```python
from build123d import *


with BuildPart() as part:
    # Sketch1 → Revolve1 (revolve)
    with BuildSketch(Plane.XY, mode=Mode.PRIVATE) as revolve1_sk:
        Polygon((-52, 0), (-52, 2), (-42, 2), (-42, 3), (42, 3), (42, 2), (52, 2), (52, 0), align=None)
    revolve(revolve1_sk.sketch.rotate(Axis((-52, 0, 0), (1, 0, 0)), 180), axis=Axis((-52, 0, 0), (1, 0, 0)))  # turned: the seam where the file's is


solid = part.part
```
Work out the finished part from the listing and answer in its coordinate system (mm). A direction names the side the tool comes from. Round coordinates to 2 decimals unless told otherwise and drop trailing zeros. Loops run counter-clockwise (first coordinate to the right, second up) from the corner with the lowest first, then second, coordinate; pieces in that order, holes last. Notation, with made-up numbers: (10, 8.25) -> (55, 8.25) arc R14 ccw to (55, 14.25) -> close; hole circle Ø8 at (-12.75, 32.5). An arc over 180 degrees is marked (long way). Write each question's results on one line, items separated by ' | '. Start each with the question number.
1. Section C-C (x = 7.5) is taken. Determine the outline of the cut face in (y, z), plus the area to 3 significant figures.
2. Find the intervals of material crossed by probe 1 along Y at (x, z) = (32.5, 0.1); probe 2 along X at (y, z) = (-2.25, 0.95); probe 3 along Y at (x, z) = (35.5, -2.4), in increasing order. Write a range as from..to.
3. Section A-A (y = 0) is taken. Determine the outline of the cut face in (x, z).
4. A tool of negligible diameter and unlimited length cuts with its end or side. For faces 1 (the face through (-47, 0, 2)), 2 (the face through (42, -1, 2)), 3 (the face through (-52, 0, 0)), from which of +Z, -Z, +X, -X, +Y, -Y can it reach the whole face along a straight path? Write none if from no direction.
5. Given pin 1 Ø2 at (x, y) = (31, 1.5) entering from -Z; pin 2 Ø1.5 at (x, z) = (-34, 2) entering from -Y; pin 3 Ø1 at (y, z) = (-0.5, -2.5) entering from -X; pin 4 Ø1.5 at (x, z) = (29, -0.5) entering from -Y, each flat-ended and moving along its own axis, determine where each tip first touches the part or whether it passes through.
6. Section D-D (x = 46) is taken. Determine the outline of the cut face in (y, z).
7. Section B-B (z = -1.15) is taken. Determine the outline of the cut face in (x, y).
Evaluation:
1) outline: circle Ø6 at (0, 0) | area: 28.3 mm2
2) probe 1: y = -3..3 | probe 2: x = -42..42 | probe 3: y = -1.8..1.8
3) outline: (-52, -2) -> (-42, -2) -> (-42, -3) -> (42, -3) -> (42, -2) -> (52, -2) -> (52, 2) -> (42, 2) -> (42, 3) -> (-42, 3) -> (-42, 2) -> (-52, 2) -> close
4) face 1: -X | face 2: +X | face 3: +Z, -Z, -X, +Y, -Y
5) pin 1: stops at z = -2.96 | pin 2: stops at y = -2.73 | pin 3: stops at x = -42 | pin 4: stops at y = -3
6) outline: circle Ø4 at (0, 0)
7) outline: (-52, -1.64) -> (-42, -1.64) -> (-42, -2.77) -> (42, -2.77) -> (42, -1.64) -> (52, -1.64) -> (52, 1.64) -> (42, 1.64) -> (42, 2.77) -> (-42, 2.77) -> (-42, 1.64) -> (-52, 1.64) -> close
